Geometry: final body of the model. Coordinates: model frame, mm. Face numbers are marked on the shaded views. A direction names the side the tool comes from. Give positions to 0.01 mm unless a question says otherwise; leave off trailing zeros. Loops run counter-clockwise (first coordinate to the right, second up) from the corner with the lowest first, then second, coordinate; pieces in that order, holes last.
from build123d import *

# Parameters (mm, degrees)
F0_W          = 303.4089505672
F0_H          = 90.0540538132
F2_DEPTH      = 76.2
F2_DEPTH_BACK = 76.2
F5_DEPTH      = 50.8
F5_DEPTH_BACK = 50.8


with BuildPart() as f2:
    # F0 (on Front) → F2 (new body, two sides)
    with BuildSketch(Plane.XZ) as f2_sk:
        with Locations((-2.6078522205, -14.2760109156)):
            Rectangle(F0_W, F0_H)
    extrude(amount=F2_DEPTH)
    extrude(f2_sk.sketch, amount=-F2_DEPTH_BACK)

    # F1 (on Front) → F3 (revolve)
    with BuildSketch(Plane.XZ):
        Polygon((57.057470793, -54.4762127101), (57.057470793, 76.3475820422), (14.8637248203, 62.2137170317), (14.8637248203, -54.4762127101), align=None)
        Polygon((57.057470793, 76.3475820422), (14.8637248203, 76.3475820422), (14.8637248203, 62.2137170317), align=None)
    revolve(axis=Axis((14.8637248203, 0, 10.935684666), (0, 0, -1)))

    # F4 (on Front) → F5 (cut, two sides)
    with BuildSketch(Plane.XZ) as f5_sk:
        Polygon((-45.7748621702, 39.0245653689), (70.5238878727, 80.0711810589), (-45.7748621702, 80.3245604038), align=None)
    extrude(amount=-F5_DEPTH, mode=Mode.SUBTRACT)
    extrude(f5_sk.sketch, amount=F5_DEPTH_BACK, mode=Mode.SUBTRACT)


solid = f2.part
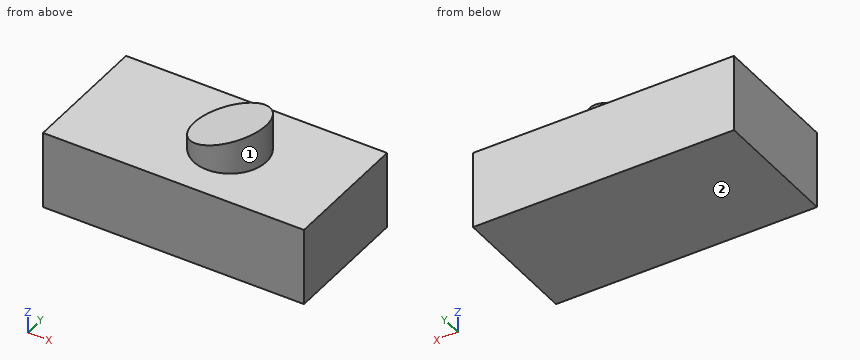
Item 1: Section query A-A on y = 0. Return loops of the section in (x, z), plus the area to 3 significant figures.
Values follow:
outline: (-154.31, -59.3) - (149.1, -59.3) - (149.1, 30.75) - (57.06, 30.75) - (57.06, 75.32) - (-27.33, 45.53) - (-27.33, 30.75) - (-154.31, 30.75) - close
area: 29,800 mm2
Item 2: Pin query (flat end, axial travel): pin 1 (1.5 mm diameter, centred on x = 16, y = -13.5, fed in from +Z); pin 2 (12 mm diameter, centred on x = 33.5, z = 42.5, fed in from +Y). Return the tip coordinate at first contact, or that it passes through.
Values follow:
pin 1: stops at z = 61.09
pin 2: stops at y = 40.26
Item 3: Section query B-B on x = 16. Return loops of the section in (y, z), plus the area to 3 significant figures.
Values follow:
outline: (-76.2, -59.3) - (76.2, -59.3) - (76.2, 30.75) - (42.18, 30.75) - (42.18, 60.83) - (-42.18, 60.83) - (-42.18, 30.75) - (-76.2, 30.75) - close
area: 16,300 mm2
Item 4: Ray query, probe 1 along Z at (x, y) = (-129, -57); probe 2 along X at (y, z) = (-31.5, 47); probe 3 along X at (y, z) = (13.5, 38). Return the intervals inside material, ascending.
Values follow:
probe 1: z = -59.3 to 30.75
probe 2: x = -13.21 to 42.94
probe 3: x = -25.11 to 54.84
Item 5: Set-up query: the marked faces 1 and 2. Return all of +Z, -Z, +X, -X, +Y, -Y with unobstructed straight access to the full face (end or side cutting, diameter ignored); none if empty.
Values follow:
face 1: +Z
face 2: -Z, +X, -X, +Y, -Y
Item 6: Section query D-D on x = -126. Return loops of the section in (y, z), plus the area to 3 significant figures.
Values follow:
outline: (-76.2, -59.3) - (76.2, -59.3) - (76.2, 30.75) - (-76.2, 30.75) - close
area: 13,700 mm2
Item 7: Section query C-C on y = 61.5. Return loops of the section in (x, z), plus the area to 3 significant figures.
Values follow:
outline: (-154.31, -59.3) - (149.1, -59.3) - (149.1, 30.75) - (-154.31, 30.75) - close
area: 27,300 mm2
